Study the drawing (mm; zero at the part's minimum x, y, z) and answer. A direction names the side the tool comes from. Round coordinates to 2 decimals unless told otherwise and drop trailing zeros. Loops run counter-clockwise (first coordinate to the right, second up) from the corner with the lowest first, then second, coordinate; pieces in that order, holes last. Notation, with made-up numbers: M 14.5,42.5 L 56.5,42.5 A7 ccw 56.5,55.5 Z; hole C 56,-29 d8. An arc over 180 degrees is marked long. Write each question's results on one line, items separated by ' | '.
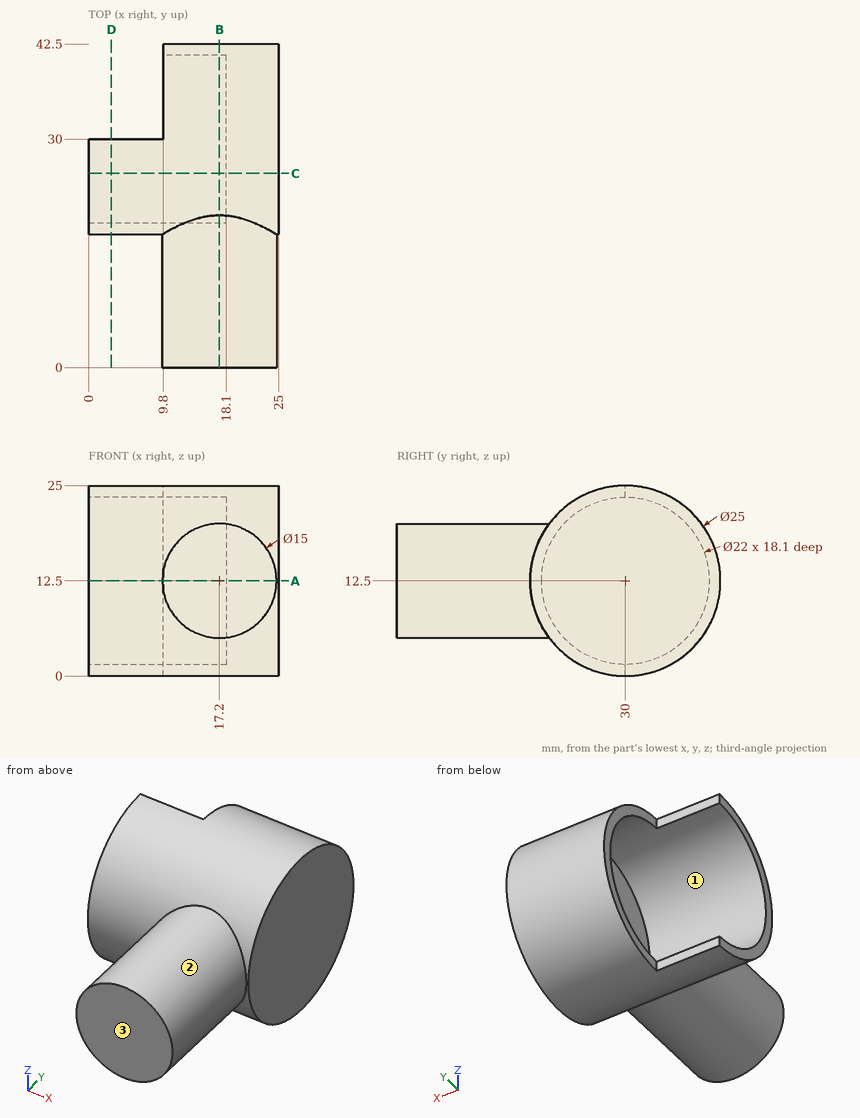
Item 1: The part is cut by section D-D (x = 3). Determine the outline of the cut face in (y, z), plus the area to 3 significant figures.
Outcome:
outline: M 30,0 L 30,1.5 A11 cw 30,23.5 L 30,25 A12.5 ccw Z | area: 55.4 mm2
Item 2: Straight lines are drawn through the part: line 1 (X direction, y = 24, z = 4); line 2 (Y direction, x = 12, z = 9.5); line 3 (Y direction, x = 10.25, z = 22). For each, find the intervals that lie inside material, in ascending order.
Outcome:
line 1: x = 18.1 to 25 | line 2: y = 0 to 19.42, 40.58 to 42.13 | line 3: y = 21.88 to 24.45, 35.55 to 38.12
Item 3: For the marked faces 1, 2 and 3, determine the directions among +Z, -Z, +X, -X, +Y, -Y from which every point of the face is accessible in a straight line to the end or side of a thin tool.
Outcome:
face 1: -X | face 2: -Y | face 3: +Z, -Z, +X, -X, -Y
Item 4: The part is cut by section C-C (y = 25.5). Determine the outline of the cut face in (x, z).
Outcome:
outline: M 0,0.84 L 25,0.84 L 25,24.16 L 0,24.16 L 0,22.54 L 18.1,22.54 L 18.1,2.46 L 0,2.46 Z
Item 5: The part is cut by section A-A (z = 12.5). Determine the outline of the cut face in (x, y).
Outcome:
outline: M 0,17.5 L 9.7,17.5 L 9.7,0 L 24.7,0 L 24.7,17.5 L 25,17.5 L 25,42.5 L 9.8,42.5 L 9.8,41 L 18.1,41 L 18.1,19 L 0,19 Z
Item 6: The part is cut by section B-B (x = 17.2). Determine the outline of the cut face in (y, z).
Outcome:
outline: M 0,5 L 20,5 A12.5 ccw long 20,20 L 0,20 Z; hole C 30,12.5 d22
Item 7: Flat-ended cylindrical pins translate along their axes: pin 1 (1 mm diameter, centred on x = 19, y = 22.5, fed in from -Z); pin 2 (1.5 mm diameter, centred on y = 30.5, z = 13.5, fed in from -X); pin 3 (14 mm diameter, centred on y = 36.5, z = 10, fed in from -X); pin 4 (1.5 mm diameter, centred on y = 19.5, z = 22, fed in from -X). Find the tip coordinate at first contact, or state that the pin passes through.
Outcome:
pin 1: stops at z = 2.14 | pin 2: stops at x = 18.1 | pin 3: stops at x = 9.8 | pin 4: passes through
